Read the model definition and answer for the solid it produces. Units are mm, in the model's axes. A direction names the side the tool comes from. Coordinates: 2 decimals unless noted, no trailing zeros. Write each loop counter-clockwise with the first axis right and the second up, starting at its lowest first coordinate (ties: lowest second). Pieces come first, ordered by that corner, then holes. Notation, with made-up numbers: (24, 21.5) -> (45, 21.5) arc R24 cw to (45, 44.5) -> close; hole circle Ø2 at (58, 76.25). An arc over 180 degrees is marked (long way). Return JSON: item names as keys, results as strings.
from build123d import *

# Parameters (mm, degrees)
BOSS_EXTRUDE1_DEPTH            = 38.1
SKETCH2_R                      = 14.2875
CUT_EXTRUDE1_DEPTH             = 39.1
F_9_0_196_DIAMETER_HOLE1_D     = 4.9784
F_9_0_196_DIAMETER_HOLE1_DEPTH = 3.175


with BuildPart() as part:
    # Sketch1 → Boss-Extrude1 (new body)
    with BuildSketch(Plane.XY):
        Polygon((-19.05, 0), (19.05, 0), (19.05, -63.5), (15.875, -63.5), (15.875, -3.175), (-15.875, -3.175), (-15.875, -63.5), (-19.05, -63.5), align=None)
    extrude(amount=BOSS_EXTRUDE1_DEPTH)

    # Sketch2 → Cut-Extrude1 (cut, through all)
    with BuildSketch(Plane(origin=(19.05, 0, 0), x_dir=(0, 0, -1), z_dir=(1, 0, 0))):
        with Locations((-19.05, -36.1499912)):
            Circle(SKETCH2_R)
    extrude(amount=-CUT_EXTRUDE1_DEPTH, mode=Mode.SUBTRACT)

    # #9 (0.196) Diameter Hole1
    with Locations(Plane(origin=(0, 0, 0), x_dir=(1, 0, 0), z_dir=(0, 1, 0))):
        with Locations((-9.525, -19.05), (9.525, -19.05)):
            Hole(F_9_0_196_DIAMETER_HOLE1_D / 2, depth=F_9_0_196_DIAMETER_HOLE1_DEPTH)


solid = part.part
1. The part is cut by section D-D (y = -47.5). Determine the outline of the cut face in (x, z) (3 decimals), then the cut area to 3 significant figures.
Taken from the geometry:
{"outline": "(-19.05, 0) -> (-15.875, 0) -> (-15.875, 10.372) -> (-19.05, 10.372) -> close; (-19.05, 27.728) -> (-15.875, 27.728) -> (-15.875, 38.1) -> (-19.05, 38.1) -> close; (15.875, 0) -> (19.05, 0) -> (19.05, 10.372) -> (15.875, 10.372) -> close; (15.875, 27.728) -> (19.05, 27.728) -> (19.05, 38.1) -> (15.875, 38.1) -> close", "area": "132 mm2"}
2. The part is cut by section A-A (y = -55.5). Determine the outline of the cut face in (x, z) (3 decimals), then the cut area to 3 significant figures.
Taken from the geometry:
{"outline": "(-19.05, 0) -> (-15.875, 0) -> (-15.875, 38.1) -> (-19.05, 38.1) -> close; (15.875, 0) -> (19.05, 0) -> (19.05, 38.1) -> (15.875, 38.1) -> close", "area": "242 mm2"}
3. The part is cut by section B-B (z = 19.05). Count the separate pieces of the cut face and the enclosed holes in it, then the cut area to 3 significant figures.
Taken from the geometry:
{"separate pieces": "5", "enclosed holes": "0", "area": "291 mm2"}
4. A tool of negligible diameter and unlimited length cuts with its end or side. For faces 1 (the face through (17.48, -24.1, 11.37)), 2 (the face through (15.875, -20, 19)), from which of +Z, -Z, +X, -X, +Y, -Y can it reach the whole face along a straight path? Write none if from no direction.
Taken from the geometry:
{"face 1": "+X, -X", "face 2": "+Z, -Z, -Y"}
5. For a pull along Z with two mould halves and no side action, classify faces 3 (the face through (0, -3.175, 19)), 4 (the face through (11.36, -1.61, 17.37)), 5 (the face through (17, -27, 38.1)) as +Z half, -Z half, draft (parallel to the pull), parting line (faces both ways), or undercut.
Taken from the geometry:
{"face 3": "draft", "face 4": "undercut", "face 5": "+Z half"}
6. The part is cut by section C-C (z = 3). Determine the outline of the cut face in (x, y) (3 decimals).
Taken from the geometry:
{"outline": "(-19.05, -63.5) -> (-15.875, -63.5) -> (-15.875, -3.175) -> (15.875, -3.175) -> (15.875, -63.5) -> (19.05, -63.5) -> (19.05, 0) -> (-19.05, 0) -> close"}
7. A flat-ended cylindrical pin translates along its axis: pin 1 Ø8 at (x, z) = (-4.5, 4.5) entering from -Y (3 decimals). Find the tip coordinate at first contact, or state that the pin passes through.
Taken from the geometry:
{"pin 1": "stops at y = -3.175"}
8. Consider L1, parallel to X at y = -1.4, z = 19.05; L2, parallel to X at y = -20.5, z = 8.5 (3 decimals); L3, parallel to Y at x = -17, z = 19. Determine where each line is inside the solid, lowest interval first.
Taken from the geometry:
{"L1": "x = -19.05 to -12.01, -7.04 to 7.04, 12.01 to 19.05", "L2": "x = -19.05 to -15.875, 15.875 to 19.05", "L3": "y = -63.5 to -50.44, -21.86 to 0"}
